Geometry: final body of the model. Coordinates: model frame, mm. Face numbers are marked on the shaded views. Give positions to 0.01 mm unless a question says otherwise; leave off trailing zeros. Write each loop counter-clockwise with the first axis right and the second up, starting at its lowest first coordinate (ties: lowest second). Pieces come first, ordered by that corner, then holes.
Q1. Section C-C (x = 22). Return the cut outline in (y, z) (3 decimals), plus the area to 3 significant figures.
Q2. Mould query, pull axis X, two halves, no side actions, for the marked faces 1 and 2. Classes: +X half, -X half, draft (parallel to the pull), parting line (faces both ways), or undercut.
Q3. Section A-A (x = -56.5). Return the cut outline in (y, z) (1 decimal).
Q4. Pin query (flat end, axial travel): pin 1 Ø4 at (y, z) = (-7.5, 5) entering from -X; pin 2 Ø2.5 at (x, y) = (50.292, 8.763) entering from +Z; pin 3 Ø1.9 at (x, z) = (-30, 3.5) entering from -Y (3 decimals); pin 4 Ø5 at (x, y) = (48.5, -4) entering from +Z. Return the tip coordinate at first contact, or that it passes through.
Q5. Line query: line 1 (Y direction, x = 49, z = 3.5) (3 decimals); line 2 (X direction, y = -10, z = 3.25); line 3 (Y direction, x = -20, z = 5) (3 decimals). Output: solid intervals per line, ascending.
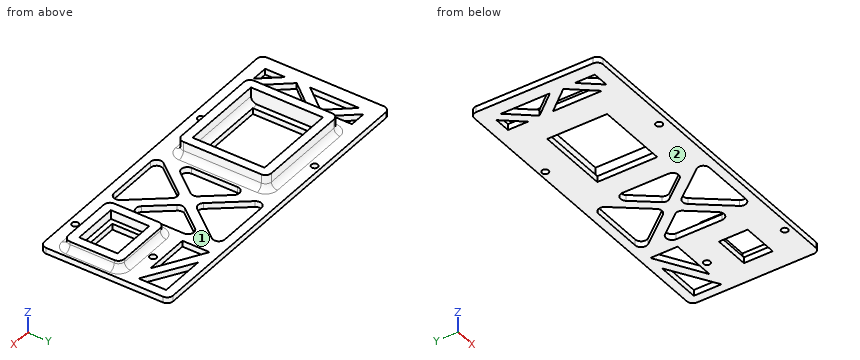
from build123d import *

# Parameters (mm, degrees)
F0_W     = 134.62
F0_H     = 54.61
F1_DEPTH = 2.54
F2_R     = 1.397
F3_DEPTH = 2.541
F2_W     = 43.18
F2_H     = 38.1
F2_W_2   = 35.56
F2_H_2   = 30.48
F4_DEPTH = 6.35
F2_W_3   = 26.924
F2_H_3   = 23.876
F2_W_4   = 19.304
F2_H_4   = 16.256
F5_DEPTH = 3.81
F6_W     = 30.48
F6_H     = 25.4
F6_W_2   = 15.24
F6_H_2   = 12.192
F7_DEPTH = 2.541
F8_R     = 2.53999
F9_R     = 2.54


# Not quite as in the source:
# - a fillet or chamfer is up to 0.001 mm smaller than in the source, because OpenCascade refuses the exact size
# - a feature names something its author has since deleted; it is built from what else it names


with BuildPart() as f1:
    # F0 (on Top) → F1 (new body)
    with BuildSketch(Plane.XY):
        Rectangle(F0_W, F0_H)
    extrude(amount=-F1_DEPTH)

    # F2 (on face) → F3 (cut, through all)
    with BuildSketch(Plane.XY):
        with Locations((-25.146, 24.765)):
            Circle(F2_R)
        with Locations((-25.146, -23.495)):
            Circle(F2_R)
        with Locations((50.292, 8.763)):
            Circle(F2_R)
        with Locations((50.292, -24.257)):
            Circle(F2_R)
    extrude(amount=-F3_DEPTH, mode=Mode.SUBTRACT)

    # F2 (on face) → F4 (join)
    with BuildSketch(Plane.XY):
        with Locations((-25.146, 0.635)):
            Rectangle(F2_W, F2_H)
        with Locations((-25.146, 0.635)):
            Rectangle(F2_W_2, F2_H_2, mode=Mode.SUBTRACT)
    extrude(amount=F4_DEPTH)

    # F2 (on face) → F5 (join)
    with BuildSketch(Plane.XY):
        with Locations((50.292, -7.747)):
            Rectangle(F2_W_3, F2_H_3)
        with Locations((50.292, -7.747)):
            Rectangle(F2_W_4, F2_H_4, mode=Mode.SUBTRACT)
    extrude(amount=F5_DEPTH)

    # F6 (on face) → F7 (cut, through all)
    with BuildSketch(Plane.XY):
        Polygon((13.7795, 0), (0.254, 17.0379360465), (0.254, -17.0379360465), align=None)
        Polygon((33.02, 23.495), (0.254, 23.495), (16.637, 2.8575), align=None)
        Polygon((33.02, -17.0379360465), (33.02, 17.0379360465), (19.4945, 0), align=None)
        Polygon((16.637, -2.8575), (0.254, -23.495), (33.02, -23.495), align=None)
        Polygon((56.3291969075, 11.811), (36.83, 23.3617037719), (36.83, 11.811), align=None)
        Polygon((63.5, 23.495), (44.0803815263, 23.495), (63.5, 11.811), align=None)
        with Locations((-25.146, 0.635)):
            Rectangle(F6_W, F6_H)
        with Locations((50.292, -7.747)):
            Rectangle(F6_W_2, F6_H_2)
        Polygon((-53.0180806356, 7.8316666667), (-61.595, 18.202451519), (-61.595, -2.5391181857), align=None)
        Polygon((-52.451, 21.59), (-59.4524328779, 21.59), (-52.451, 13.1242151477), align=None)
        Polygon((-52.451, -18.202451519), (-52.451, 2.5391181857), (-61.0279193644, -7.8316666667), align=None)
        Polygon((-54.5935671221, -21.59), (-61.595, -13.1242151477), (-61.595, -21.59), align=None)
    extrude(amount=-F7_DEPTH, mode=Mode.SUBTRACT)

    # F8 (radius 2.54 in the source; OpenCascade refuses exactly that, so slightly less here)
    f8_edges = [f1.edges().sort_by_distance(p)[0] for p in [
        (-25.146, -18.415, 0),
        (-46.736, 0.635, 0),
        (50.292, -19.685, 0),
        (36.83, -7.747, 0),
        (-25.146, 19.685, 0),
        (-3.556, 0.635, 0),
        (63.754, -7.747, 0),
        (50.292, 4.191, 0),
        (63.754, 4.191, 1.905),
        (63.754, -19.685, 1.905),
        (-3.556, 19.685, 3.175),
        (-3.556, -18.415, 3.175),
        (36.83, -19.685, 1.905),
        (-46.736, -18.415, 3.175),
        (-46.736, 19.685, 3.175),
        (36.83, 4.191, 1.905),
        (-25.146, 15.875, 0),
        (-25.146, -14.605, 0),
        (-67.31, -27.305, -1.27),
        (-67.31, 27.305, -1.27),
        (67.31, 27.305, -1.27),
        (67.31, -27.305, -1.27),
    ]]
    fillet(f8_edges, radius=F8_R)

    # F9
    f9_edges = [f1.edges().sort_by_distance(p)[0] for p in [
        (33.02, 23.495, -1.27),
        (13.7795, 0, -1.27),
        (16.637, -2.8575, -1.27),
        (0.254, 17.037936, -1.27),
        (33.02, 17.037936, -1.27),
        (33.02, -17.037936, -1.27),
        (33.02, -23.495, -1.27),
        (0.254, 23.495, -1.27),
        (0.254, -23.495, -1.27),
        (0.254, -17.037936, -1.27),
        (19.4945, 0, -1.27),
        (16.637, 2.8575, -1.27),
    ]]
    fillet(f9_edges, radius=F9_R)


solid = f1.part
Computed:
1. outline: (-27.305, -2.54) - (-23.495, -2.54) - (-23.495, 0) - (-27.305, 0) - close; (-9.613, -2.54) - (-3.156, -2.54) - (-3.156, 0) - (-9.613, 0) - close; (3.156, -2.54) - (9.613, -2.54) - (9.613, 0) - (3.156, 0) - close; (23.495, -2.54) - (27.305, -2.54) - (27.305, 0) - (23.495, 0) - close
1. area: 52.2 mm2
2. face 1: undercut
2. face 2: draft
3. outline: (-27.3, -2.5) - (-21.6, -2.5) - (-21.6, 0) - (-27.3, 0) - close; (-19.3, -2.5) - (-13.3, -2.5) - (-13.3, 0) - (-19.3, 0) - close; (-2.4, -2.5) - (3.6, -2.5) - (3.6, 0) - (-2.4, 0) - close; (12, -2.5) - (18, -2.5) - (18, 0) - (12, 0) - close; (21.6, -2.5) - (27.3, -2.5) - (27.3, 0) - (21.6, 0) - close
4. pin 1: stops at x = -46.74
4. pin 2: passes through
4. pin 3: stops at y = -18.415
4. pin 4: stops at z = 0
5. line 1: y = -19.685 to -15.875, 0.381 to 4.191
5. line 2: x = -46.74 to -42.93, -7.37 to -3.56, 36.83 to 40.64, 59.94 to 63.75
5. line 3: y = -18.415 to -14.605, 15.875 to 19.685
